Design review of the part shown in the three views and the two pictorial views. Dimensions are in mm from the part's minimum x, y and z. Give positions to 0.01 mm unless a question says otherwise; leave off trailing zeros. Order: outer loops, then holes, each group sorted by start corner. A loop starts at its lowest first (then second) coordinate and runs counter-clockwise, first axis right, second up.
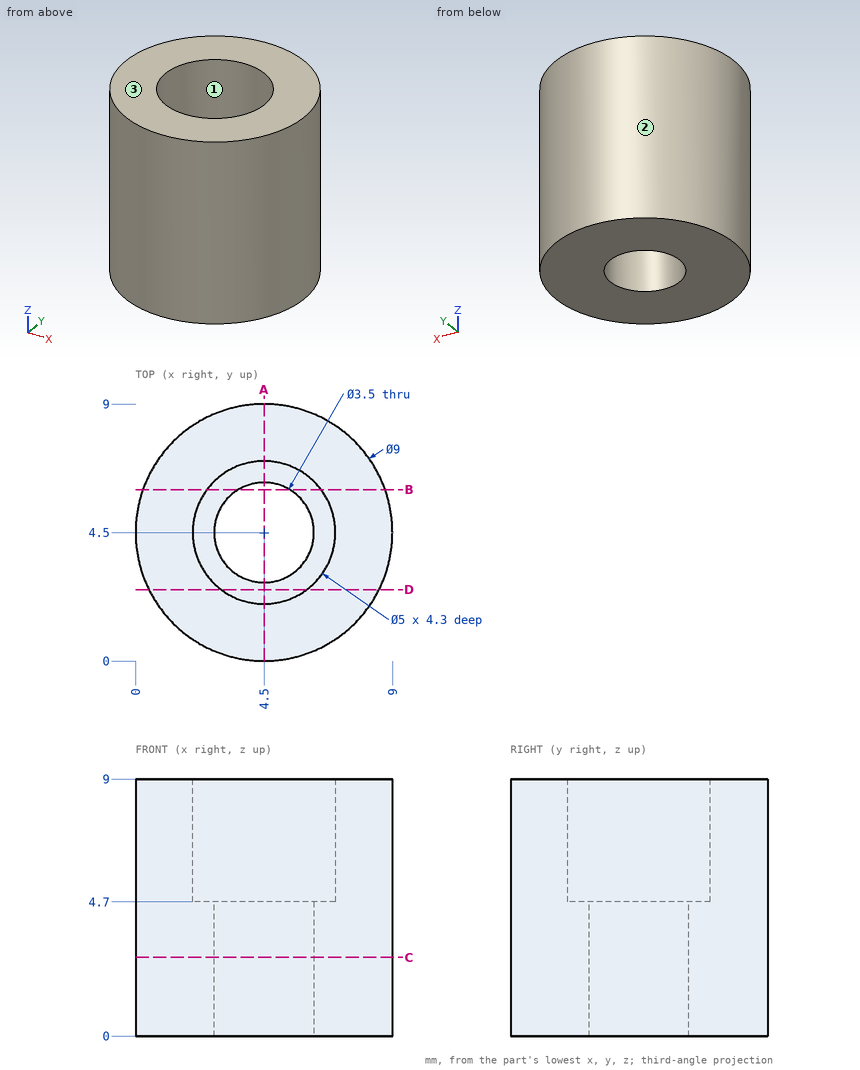
Item 1: For line 1 (Y direction, x = 4.5, z = 3.2); line 2 (Y direction, x = 4.5, z = 7.6); line 3 (Z direction, x = 5.75, y = 6), list the stretches that pass through material, from the lowest coordinate up.
Values found:
line 1: y = 0 to 2.75, 6.25 to 9
line 2: y = 0 to 2, 7 to 9
line 3: z = 0 to 4.7
Item 2: Draft analysis for pull direction Y (two halves, no side actions). For the marked faces 1, 2 and 3, state which applies: released by +Y, released by -Y, zero draft, split by the parting line, or undercut.
Values found:
face 1: undercut
face 2: split by the parting line
face 3: zero draft
Item 3: Take a section at D-D (y = 2.5). Give the boundary of the cut face in (x, z).
Values found:
outline: (0.47, 0) - (8.53, 0) - (8.53, 9) - (6, 9) - (6, 4.7) - (3, 4.7) - (3, 9) - (0.47, 9) - close
Item 4: Take a section at B-B (y = 6). Give the boundary of the cut face in (x, z).
Values found:
outline: (0.26, 0) - (3.6, 0) - (3.6, 4.7) - (2.5, 4.7) - (2.5, 9) - (0.26, 9) - close; (5.4, 0) - (8.74, 0) - (8.74, 9) - (6.5, 9) - (6.5, 4.7) - (5.4, 4.7) - close
Item 5: Take a section at A-A (x = 4.5). Give the boundary of the cut face in (y, z), and give its area (4 significant figures).
Values found:
outline: (0, 0) - (2.75, 0) - (2.75, 4.7) - (2, 4.7) - (2, 9) - (0, 9) - close; (6.25, 0) - (9, 0) - (9, 9) - (7, 9) - (7, 4.7) - (6.25, 4.7) - close
area: 43.05 mm2
Item 6: Clearance check with flat-ended pins moving along their axes: pin 1 Ø4 at (y, z) = (7, 4) entering from -X; pin 2 Ø3 at (y, z) = (4, 1.5) entering from +X; pin 3 Ø1 at (x, z) = (1, 2.5) entering from +Y; pin 4 Ø1.5 at (x, z) = (2, 4.5) entering from -Y. State where each tip first meets the part, or that it passes through.
Values found:
pin 1: stops at x = 0.03
pin 2: stops at x = 9
pin 3: stops at y = 7.85
pin 4: stops at y = 0.35
Item 7: Take a section at C-C (z = 2.75). Give the boundary of the cut face in (x, y).
Values found:
outline: circle Ø9 at (4.5, 4.5); hole circle Ø3.5 at (4.5, 4.5)
